Can you work these out from the model? Positions are in its coordinate system, mm. Face numbers are marked on the shaded views. A direction names the side the tool comes from. Give positions to 0.01 mm unless a question says otherwise; leave off trailing zeros. Order: outer loops, then holes, each group sorted by start corner. A loop starts at its lowest first (then second) coordinate and runs counter-clockwise, first axis right, second up. Notation, with made-up numbers: (-13.75, 14) - (20.25, 14) arc R16 ccw to (20.25, 32) - close; hole circle Ø1 at (-9.75, 4.25). An arc over 180 degrees is marked (long way). Return JSON: item names as keys, results as strings.
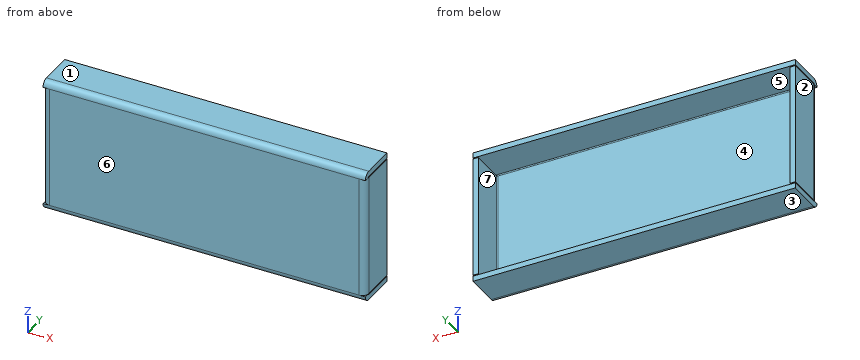
```python
from build123d import *

# Parameters (mm, degrees)
CROQUIS2_W                         = 240
CROQUIS2_H                         = 100
BRIDA_BASE1_DEPTH                  = 4
BRIDA_DE_ARISTA1_STRIP_W           = 17.4732
BRIDA_DE_ARISTA1_STRIP_H           = 4
BRIDA_DE_ARISTA1_STRIP_CUT_DEPTH   = 240
BRIDA_DE_ARISTA1_STRIP_2_W         = 17.4732
BRIDA_DE_ARISTA1_STRIP_2_H         = 4
BRIDA_DE_ARISTA1_STRIP_CUT_2_DEPTH = 240
BRIDA_DE_ARISTA1_DEPTH             = 240
BRIDA_DE_ARISTA1_BEND_DEPTH        = 240
BRIDA_DE_ARISTA2_STRIP_W           = 17.4732
BRIDA_DE_ARISTA2_STRIP_H           = 4
BRIDA_DE_ARISTA2_STRIP_CUT_DEPTH   = 90.5268
BRIDA_DE_ARISTA2_STRIP_2_W         = 17.4732
BRIDA_DE_ARISTA2_STRIP_2_H         = 4
BRIDA_DE_ARISTA2_STRIP_CUT_2_DEPTH = 90.5268
BRIDA_DE_ARISTA2_DEPTH             = 90.5268
BRIDA_DE_ARISTA2_BEND_DEPTH        = 90.5268


# Sheet-metal steps are written as plain solids
with BuildPart() as part:
    # Croquis2 → Brida base1 (new body)
    with BuildSketch(Plane(origin=(0, 0, 0), x_dir=(1, 0, 0), z_dir=(0, 1, 0))):
        with Locations((120, 50)):
            Rectangle(CROQUIS2_W, CROQUIS2_H)
    extrude(amount=BRIDA_BASE1_DEPTH)

    # Brida de arista1 strip (across the edge) → Brida de arista1 strip cut (cut)
    with BuildSketch(Plane(origin=(0, 4, 0), x_dir=(0, 0, -1), z_dir=(1, 0, 0))):
        with Locations((-4, -2)):
            Rectangle(BRIDA_DE_ARISTA1_STRIP_W, BRIDA_DE_ARISTA1_STRIP_H)
    extrude(amount=BRIDA_DE_ARISTA1_STRIP_CUT_DEPTH, mode=Mode.SUBTRACT)

    # Brida de arista1 strip 2 (across the edge) → Brida de arista1 strip cut 2 (cut)
    with BuildSketch(Plane(origin=(240, 4, -100), x_dir=(0, 0, 1), z_dir=(-1, 0, 0))):
        with Locations((-4, -2)):
            Rectangle(BRIDA_DE_ARISTA1_STRIP_2_W, BRIDA_DE_ARISTA1_STRIP_2_H)
    extrude(amount=BRIDA_DE_ARISTA1_STRIP_CUT_2_DEPTH, mode=Mode.SUBTRACT)

    # Brida de arista1 section (across the edge) → Brida de arista1 (add)
    with BuildSketch(Plane(origin=(0, 4, 0), x_dir=(0, 0, -1), z_dir=(1, 0, 0))):
        with BuildLine():
            Line((0, 0.7366), (0, 26))
            Line((0, 26), (4, 26))
            Line((4, 26), (4, 0.7366))
            ThreePointArc((4, 0.7366), (4.215745145, 0.215745145), (4.7366, 0))
            Line((4.7366, 0), (4.7366, -4))
            ThreePointArc((4.7366, -4), (1.38731802, -2.61268198), (0, 0.7366))
        make_face()
    extrude(amount=BRIDA_DE_ARISTA1_DEPTH)

    # Brida de arista1 section 2 (across the edge) → Brida de arista1 bend (add)
    with BuildSketch(Plane(origin=(240, 4, -100), x_dir=(0, 0, 1), z_dir=(-1, 0, 0))):
        with BuildLine():
            Line((0, 0.7366), (0, 26))
            Line((0, 26), (4, 26))
            Line((4, 26), (4, 0.7366))
            ThreePointArc((4, 0.7366), (4.215745145, 0.215745145), (4.7366, 0))
            Line((4.7366, 0), (4.7366, -4))
            ThreePointArc((4.7366, -4), (1.38731802, -2.61268198), (0, 0.7366))
        make_face()
    extrude(amount=BRIDA_DE_ARISTA1_BEND_DEPTH)

    # Brida de arista2 strip (across the edge) → Brida de arista2 strip cut (cut)
    with BuildSketch(Plane(origin=(240, 4, -4.7366), x_dir=(-1, 0, 0), z_dir=(0, 0, -1))):
        with Locations((-4, -2)):
            Rectangle(BRIDA_DE_ARISTA2_STRIP_W, BRIDA_DE_ARISTA2_STRIP_H)
    extrude(amount=BRIDA_DE_ARISTA2_STRIP_CUT_DEPTH, mode=Mode.SUBTRACT)

    # Brida de arista2 strip 2 (across the edge) → Brida de arista2 strip cut 2 (cut)
    with BuildSketch(Plane(origin=(0, 4, -95.2634), x_dir=(1, 0, 0), z_dir=(0, 0, 1))):
        with Locations((-4, -2)):
            Rectangle(BRIDA_DE_ARISTA2_STRIP_2_W, BRIDA_DE_ARISTA2_STRIP_2_H)
    extrude(amount=BRIDA_DE_ARISTA2_STRIP_CUT_2_DEPTH, mode=Mode.SUBTRACT)

    # Brida de arista2 section (across the edge) → Brida de arista2 (add)
    with BuildSketch(Plane(origin=(240, 4, -4.7366), x_dir=(-1, 0, 0), z_dir=(0, 0, -1))):
        with BuildLine():
            Line((0, 0.7366), (0, 26))
            Line((0, 26), (4, 26))
            Line((4, 26), (4, 0.7366))
            ThreePointArc((4, 0.7366), (4.215745145, 0.215745145), (4.7366, 0))
            Line((4.7366, 0), (4.7366, -4))
            ThreePointArc((4.7366, -4), (1.38731802, -2.61268198), (0, 0.7366))
        make_face()
    extrude(amount=BRIDA_DE_ARISTA2_DEPTH)

    # Brida de arista2 section 2 (across the edge) → Brida de arista2 bend (add)
    with BuildSketch(Plane(origin=(0, 4, -95.2634), x_dir=(1, 0, 0), z_dir=(0, 0, 1))):
        with BuildLine():
            Line((0, 0.7366), (0, 26))
            Line((0, 26), (4, 26))
            Line((4, 26), (4, 0.7366))
            ThreePointArc((4, 0.7366), (4.215745145, 0.215745145), (4.7366, 0))
            Line((4.7366, 0), (4.7366, -4))
            ThreePointArc((4.7366, -4), (1.38731802, -2.61268198), (0, 0.7366))
        make_face()
    extrude(amount=BRIDA_DE_ARISTA2_BEND_DEPTH)


solid = part.part
```
1. For pin 1 Ø1.5 at (x, z) = (194, -44.5) entering from +Y; pin 2 Ø4.5 at (x, y) = (2, 1) entering from -Z; pin 3 Ø3 at (x, y) = (3.5, 1.5) entering from +Z, each with a flat end and sliding along its axis, tell me the tip position at first contact or that it passes through.
Checks:
{"pin 1": "y = 4", "pin 2": "z = -99.76", "pin 3": "z = -0.33"}
2. Suppose I cut it at C-C (z = -56). List the corners of the cut face in (x, y) for me, plus the area to 3 significant figures.
Checks:
{"outline": "(0, 4.74) arc R4.74 ccw to (4.74, 0) - (235.26, 0) arc R4.74 ccw to (240, 4.74) - (240, 30) - (236, 30) - (236, 4.74) arc R0.74 cw to (235.26, 4) - (4.74, 4) arc R0.74 cw to (4, 4.74) - (4, 30) - (0, 30) - close", "area": "1,160 mm^2"}
3. On a 3-axis mill with a long thin cutter (end or side, diameter ignored), from which of +Z, -Z, +X, -X, +Y, -Y can I reach the whole of each face in a straight line? I mean the marked faces 5, 6 and 7. Say none if no direction works.
Checks:
{"face 5": "+X, -X, +Y", "face 6": "+Z, -Z, +X, -X, -Y", "face 7": "+Y"}
4. Thinking about a two-plate mould opening in Z: for the marked faces 1, 2, 3 and 4, which applies, +Z half, -Z half, draft (parallel to the pull), parting line (faces both ways), or undercut?
Checks:
{"face 1": "+Z half", "face 2": "draft", "face 3": "-Z half", "face 4": "undercut"}
5. Suppose I cut it at B-B (x = 60). List the corners of the cut face in (y, z) for me.
Checks:
{"outline": "(0, -95.26) arc R4.74 ccw to (4.74, -100) - (30, -100) - (30, -96) - (4.74, -96) arc R0.74 cw to (4, -95.26) - (4, -4.74) arc R0.74 cw to (4.74, -4) - (30, -4) - (30, 0) - (4.74, 0) arc R4.74 ccw to (0, -4.74) - close"}
6. Suppose I cut it at A-A (y = 25.25). List the corners of the cut face in (x, z) for me.
Checks:
{"outline": "(0, -100) - (240, -100) - (240, -96) - (0, -96) - close; (0, -95.26) - (4, -95.26) - (4, -4.74) - (0, -4.74) - close; (0, -4) - (240, -4) - (240, 0) - (0, 0) - close; (236, -95.26) - (240, -95.26) - (240, -4.74) - (236, -4.74) - close"}
7. If I drill on L1, parallel to X at y = 28.75, z = -77; L2, parallel to Z at x = 47, y = 21; L3, parallel to Y at x = 41.5, z = -88.5, over which ranges is the centre line in solid material (lowest first)? Write a range as [from, to].
Checks:
{"L1": "[0, 4], [236, 240]", "L2": "[-100, -96], [-4, 0]", "L3": "[0, 4]"}
